For this review, take the finished solid that the model builds, in its own axes (mm). Give positions to 0.01 mm unless a question says otherwise; leave off trailing zeros. Order: outer loops, then holes, each group sorted by start corner. A loop starts at its lowest first (then second) coordinate and runs counter-clockwise, first axis right, second up. Notation, with made-up numbers: (-23, 45) -> (34, 45) arc R15 cw to (34, 69) -> close; hole circle Ø11 at (54.5, 14). An arc over 180 degrees is marked (long way). Return JSON: item names as keys, results as strings. Group by question number.
1) Add section D-D (x = 1.05). State how many separate pieces and enclosed holes the cut face has, then the cut area to 3 significant figures.
2) Insertion check: P1, Ø1.5, axis at y = -8.5, z = 4.5, coming from the -X side; P2, Ø1.5, axis at x = 2.5, y = 12.5, coming from the +Z side; P3, Ø3, axis at y = 6.45, z = 3.72, coming from the +X side; P4, Ø1.5, axis at x = 0.5, y = 14, coming from the -Z side. Each pin has a flat end and moves straight along its axis. Give the tip position at first contact, or say it passes through.
3) Add section B-B (y = 0). Give the boundary of the cut face in (x, z) (1 decimal), then the cut area to 3 significant figures.
4) Add section C-C (y = 5.5). Give the boundary of the cut face in (x, z) (3 decimals).
5) To check wall thickness, follow line 1 along Z through (x, y) = (1.2, -7.5); line 2 along Y through (x, z) = (1.45, -5); line 3 along Y through (x, z) = (1.25, 3). State the ranges of each line that lie inside material, in increasing order.
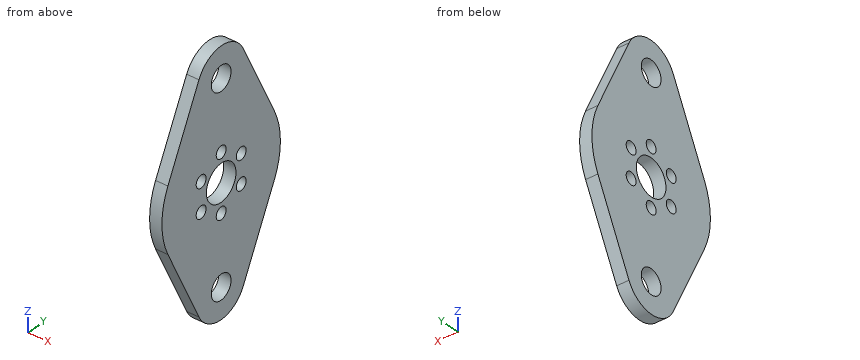
from build123d import *

# Parameters (mm, degrees)
SKETCH1_R           = 4.7625
SKETCH1_R_2         = 3.175
SKETCH1_R_3         = 1.5875
BOSS_EXTRUDE1_DEPTH = 3.175


with BuildPart() as part:
    # Sketch1 → Boss-Extrude1 (new body)
    with BuildSketch(Plane(origin=(0, 0, 0), x_dir=(0, 0, -1), z_dir=(1, 0, 0))):
        with BuildLine():
            Line((-28.87265625, 7.137546134), (-8.334375, 17.130110722))
            ThreePointArc((-8.334375, 17.130110722), (0, 19.05), (8.334375, 17.130110722))
            Line((8.334375, 17.130110722), (28.87265625, 7.137546134))
            ThreePointArc((28.87265625, 7.137546134), (33.3375, 0), (28.87265625, -7.137546134))
            Line((28.87265625, -7.137546134), (8.334375, -17.130110722))
            ThreePointArc((8.334375, -17.130110722), (0, -19.05), (-8.334375, -17.130110722))
            Line((-8.334375, -17.130110722), (-28.87265625, -7.137546134))
            ThreePointArc((-28.87265625, -7.137546134), (-33.3375, 0), (-28.87265625, 7.137546134))
        make_face()
        Circle(SKETCH1_R, mode=Mode.SUBTRACT)
        with Locations((-25.4, 0)):
            Circle(SKETCH1_R_2, mode=Mode.SUBTRACT)
        with Locations((25.4, 0)):
            Circle(SKETCH1_R_2, mode=Mode.SUBTRACT)
        with Locations((-3.7211, -6.44513426)):
            Circle(SKETCH1_R_3, mode=Mode.SUBTRACT)
        with Locations((3.7211, 6.44513426)):
            Circle(SKETCH1_R_3, mode=Mode.SUBTRACT)
        with Locations((3.7211, -6.44513426)):
            Circle(SKETCH1_R_3, mode=Mode.SUBTRACT)
        with Locations((-3.7211, 6.44513426)):
            Circle(SKETCH1_R_3, mode=Mode.SUBTRACT)
        with Locations((-7.4422, 0)):
            Circle(SKETCH1_R_3, mode=Mode.SUBTRACT)
        with Locations((7.4422, 0)):
            Circle(SKETCH1_R_3, mode=Mode.SUBTRACT)
    extrude(amount=BOSS_EXTRUDE1_DEPTH)


solid = part.part
Evaluation:
{
 "1": {"separate pieces": "1", "enclosed holes": "9", "area": "1,520 mm^2"},
 "2": {"P1": "x = 0", "P2": "z = 19.39", "P3": "through", "P4": "z = -16.31"},
 "3": {"outline": "(0, -33.3) -> (3.2, -33.3) -> (3.2, -28.6) -> (0, -28.6) -> close; (0, -22.2) -> (3.2, -22.2) -> (3.2, -9) -> (0, -9) -> close; (0, -5.9) -> (3.2, -5.9) -> (3.2, -4.8) -> (0, -4.8) -> close; (0, 4.8) -> (3.2, 4.8) -> (3.2, 5.9) -> (0, 5.9) -> close; (0, 9) -> (3.2, 9) -> (3.2, 22.2) -> (0, 22.2) -> close; (0, 28.6) -> (3.2, 28.6) -> (3.2, 33.3) -> (0, 33.3) -> close", "area": "121 mm^2"},
 "4": {"outline": "(0, -31.123) -> (3.175, -31.123) -> (3.175, -4.997) -> (0, -4.997) -> close; (0, -2.446) -> (3.175, -2.446) -> (3.175, 2.446) -> (0, 2.446) -> close; (0, 4.997) -> (3.175, 4.997) -> (3.175, 31.123) -> (0, 31.123) -> close"},
 "5": {"line 1": "-28.13 to -4.91, -2.53 to 2.53, 4.91 to 28.13", "line 2": "-18.38 to -7.39, -5.5 to 5.5, 7.39 to 18.38", "line 3": "-18.81 to -7.86, -5.03 to -3.7, 3.7 to 5.03, 7.86 to 18.81"}
}
